```python
from build123d import *

# Parameters (mm, degrees)
BOSS_EXTRUDE1_DEPTH     = 20
SKETCH3_R               = 3.25
CUT_EXTRUDE1_DEPTH      = 20
CUT_EXTRUDE1_DEPTH_BACK = 20


with BuildPart() as part:
    # Sketch1 → Boss-Extrude1 (new body)
    with BuildSketch(Plane.XY):
        with BuildLine():
            Line((-44.097792079, -34.850100287), (-44.097792079, -44.850100287))
            Line((-44.097792079, -44.850100287), (15.902191644, -44.850100287))
            Line((15.902191644, -44.850100287), (15.902191644, -34.850100287))
            Line((15.902191644, -34.850100287), (5.481837679, -34.850100287))
            ThreePointArc((5.481837679, -34.850100287), (3.860980617, -34.374545252), (2.753994712, -33.098648543))
            Line((2.753994712, -33.098648543), (-35.815277858, 51.167953451))
            Line((-35.815277858, 51.167953451), (-35.815277858, 60.291959238))
            Line((-35.815277858, 60.291959238), (-33.576612404, 60.291959238))
            Line((-33.576612404, 60.291959238), (-33.576612404, 62.924734339))
            Line((-33.576612404, 62.924734339), (-40.180850679, 62.924734339))
            Line((-40.180850679, 62.924734339), (-42.770369484, 68.117950349))
            ThreePointArc((-42.770369484, 68.117950349), (-44.613967183, 70.138587546), (-47.244946047, 70.886770262))
            Line((-47.244946047, 70.886770262), (-57.300660313, 70.886770262))
            ThreePointArc((-57.300660313, 70.886770262), (-60.906449606, 69.350624123), (-62.296631179, 65.686083691))
            Line((-62.296631179, 65.686083691), (-61.293211228, 40.706550479))
            ThreePointArc((-61.293211228, 40.706550479), (-60.463803823, 37.168602153), (-58.148414135, 34.367894102))
            Line((-58.148414135, 34.367894102), (-47.87808719, 26.565161379))
            Line((-47.87808719, 26.565161379), (-24.43830161, -29.850100287))
            ThreePointArc((-24.43830161, -29.850100287), (-25.902767704, -33.385634193), (-29.43830161, -34.850100287))
            Line((-29.43830161, -34.850100287), (-35.915534593, -34.850100287))
            Line((-35.915534593, -34.850100287), (-44.097792079, -34.850100287))
        make_face()
    extrude(amount=BOSS_EXTRUDE1_DEPTH)

    # Sketch3 → Cut-Extrude1 (cut, two sides)
    with BuildSketch(Plane(origin=(0, -34.850100287, 0), x_dir=(1, 0, 0), z_dir=(0, 1, 0))) as cut_extrude1_sk:
        with Locations((9.902191644, -10)):
            Circle(SKETCH3_R)
        with Locations((-36.038433316, -10)):
            Circle(SKETCH3_R)
    extrude(amount=CUT_EXTRUDE1_DEPTH, mode=Mode.SUBTRACT)
    extrude(cut_extrude1_sk.sketch, amount=-CUT_EXTRUDE1_DEPTH_BACK, mode=Mode.SUBTRACT)


solid = part.part
```
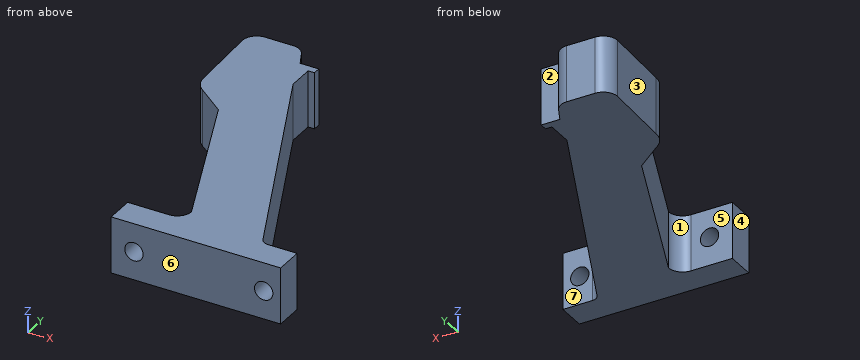
Could you check a few things on this model? Use its own coordinates, in mm. Face numbers are marked on the shaded views. A direction names the side the tool comes from. Coordinates: 2 decimals unless noted, no trailing zeros. Order: outer loops, then holes, each group sorted by start corner. A loop starts at its lowest first (then second) coordinate and runs counter-clockwise, first axis right, second up. Notation, with made-up numbers: M 19.5,47.25 L 47.5,47.25 A18 cw 47.5,68.25 Z; hole C 61,62 d3. An arc over 180 degrees is marked long. Use one line per item in the form item = value. Start each with the question number.
1. Suppose I cut it at B-B on x = 8. Write out the boundary of the cut face in (y, z), then the cut area to 3 significant figures.
2. Suppose I cut it at A-A on z = 4.75. Write out the boundary of the cut face in (x, y), then the cut area to 3 significant figures.
3. We'd pull the mould along Y, two halves only. Please class the marked faces 1, 2, 3 and 4: +Y half, -Y half, draft (parallel to the pull), parting line (faces both ways), or undercut.
4. Suppose I cut it at D-D on x = -9.5. Write out the boundary of the cut face in (y, z).
5. On a 3-axis mill with a long thin cutter (end or side, diameter ignored), from which of +Z, -Z, +X, -X, +Y, -Y can I reach the whole of each face in a straight line? I mean the marked faces 5, 6 and 7. Say none if no direction works.
6. Please list where these lines run through material, in increasing order: line 1 (X direction, y = -42.25, z = 10); line 2 (X direction, y = -39, z = 12.25); line 3 (Y direction, x = -43.5, z = 5).
7. Suppose I cut it at C-C on y = -20. Write out the boundary of the cut face in (x, z), then the cut area to 3 significant figures.
8. For pin 1 (5 mm diameter, centred on x = 13, z = 6.5, fed in from +Y); pin 2 (10 mm diameter, centred on y = 53.5, z = 10.5, fed in from +X); pin 3 (8 mm diameter, centred on y = 7, z = 11.5, fed in from -X), each with a flat end and sliding along its axis, tell me the tip position at first contact or that it passes through.
Geometry says:
q1.outline = M -44.85,0 L -34.85,0 L -34.85,7.36 L -44.85,7.36 Z; M -44.85,12.64 L -34.85,12.64 L -34.85,20 L -44.85,20 Z
q1.area = 147 mm^2
q2.outline = M -62.3,65.69 L -61.29,40.71 A7.96 ccw -58.15,34.37 L -47.88,26.57 L -24.44,-29.85 A5 cw -29.44,-34.85 L -44.1,-34.85 L -44.1,-44.85 L 15.9,-44.85 L 15.9,-34.85 L 5.48,-34.85 A3 cw 2.75,-33.1 L -35.82,51.17 L -35.82,60.29 L -33.58,60.29 L -33.58,62.92 L -40.18,62.92 L -42.77,68.12 A5 ccw -47.24,70.89 L -57.3,70.89 A5 ccw Z
q2.area = 3,290 mm^2
q3.face_1 = undercut
q3.face_2 = +Y half
q3.face_3 = -Y half
q3.face_4 = draft
q4.outline = M -44.85,0 L -6.33,0 L -6.33,20 L -44.85,20 Z
q5.face_5 = +Z, -Z, -X
q5.face_6 = +Z, -Z, +X, -X, -Y
q5.face_7 = +Z, -Z, +X, +Y
q6.line_1 = -44.1 to -39.29, -32.79 to 6.65, 13.15 to 15.9
q6.line_2 = -44.1 to -38.38, -33.69 to 7.56, 12.25 to 15.9
q6.line_3 = -44.85 to -34.85, 16.03 to 69.2
q7.outline = M -28.53,0 L -3.24,0 L -3.24,20 L -28.53,20 Z
q7.area = 506 mm^2
q8.pin_1 = -34.85
q8.pin_2 = -34.59
q8.pin_3 = -41.41
